```python
from build123d import *

# Parameters (mm, degrees)
MODEL_R                 = 1.5
SALIENTE_EXTRUIR1_DEPTH = 3


with BuildPart() as part:
    # Model → Saliente-Extruir1 (new body)
    with BuildSketch(Plane.XY):
        with BuildLine():
            Line((213.25077615, 152.428489513), (213.25077615, 188.428489513))
            ThreePointArc((213.25077615, 188.428489513), (208.75077615, 192.928489513), (204.25077615, 188.428489513))
            Line((204.25077615, 188.428489513), (204.25077615, 152.428489513))
            ThreePointArc((204.25077615, 152.428489513), (208.75077615, 147.928489513), (213.25077615, 152.428489513))
        make_face()
        with Locations((208.75077615, 179.428489513)):
            Circle(MODEL_R, mode=Mode.SUBTRACT)
        with Locations((208.75077615, 188.428489513)):
            Circle(MODEL_R, mode=Mode.SUBTRACT)
        with Locations((208.75077615, 152.428489513)):
            Circle(MODEL_R, mode=Mode.SUBTRACT)
        with Locations((208.75077615, 161.428489513)):
            Circle(MODEL_R, mode=Mode.SUBTRACT)
        with Locations((208.75077615, 170.428489513)):
            Circle(MODEL_R, mode=Mode.SUBTRACT)
    extrude(amount=SALIENTE_EXTRUIR1_DEPTH)


solid = part.part
```
For this review, take the finished solid that the model builds, in its own axes (mm). Give positions to 0.01 mm unless a question says otherwise; leave off trailing zeros. Write each loop counter-clockwise with the first axis right and the second up, starting at its lowest first coordinate (ties: lowest second). Pieces come first, ordered by that corner, then holes. Notation, with made-up numbers: M 71.25,64.5 L 128.25,64.5 A34 ccw 128.25,96.5 Z; hole C 62,72 d9. An arc over 180 degrees is marked long. One line per item, written item: value.
1) Take a section at C-C, the plane z = 1.45. Write out the cut boundary in (x, y), then the cut area to 3 significant figures.
Results are:
outline: M 204.25,152.43 A4.5 ccw 213.25,152.43 L 213.25,188.43 A4.5 ccw 204.25,188.43 Z; hole C 208.75,152.43 d3; hole C 208.75,161.43 d3; hole C 208.75,170.43 d3; hole C 208.75,179.43 d3; hole C 208.75,188.43 d3
area: 352 mm²
2) Take a section at B-B, the plane y = 153. Write out the cut boundary in (x, z).
Results are:
outline: M 204.25,0 L 207.36,0 L 207.36,3 L 204.25,3 Z; M 210.14,0 L 213.25,0 L 213.25,3 L 210.14,3 Z
3) For line 1 (X direction, y = 152.5, z = 0.2); line 2 (Y direction, x = 209, z = 0.4); line 3 (X direction, y = 160.5, z = 2.55), list the stretches that pass through material, from the lowest coordinate up. Write a range as from..to.
Results are:
line 1: x = 204.25..207.25, 210.25..213.25
line 2: y = 147.94..150.95, 153.91..159.95, 162.91..168.95, 171.91..177.95, 180.91..186.95, 189.91..192.92
line 3: x = 204.25..207.57, 209.93..213.25
4) The part is to be moulded in two halves that separate along X. For faces 1 (the flat face through (213.251, 170, 1)), 2 (the cylindrical face through (208.85, 192.927, 1.479)), 3 (the cylindrical face through (208.556, 189.916, 1.479)), say which applies: +X half, -X half, draft (parallel to the pull), parting line (faces both ways), or undercut.
Results are:
face 1: +X half
face 2: parting line
face 3: undercut
5) Take a section at D-D, the plane x = 205. Write out the cut boundary in (y, z), then the cut area to 3 significant figures.
Results are:
outline: M 149.94,0 L 190.91,0 L 190.91,3 L 149.94,3 Z
area: 123 mm²
6) Take a section at A-A, the plane x = 208. Write out the cut boundary in (y, z), then the cut area to 3 significant figures.
Results are:
outline: M 147.99,0 L 151.13,0 L 151.13,3 L 147.99,3 Z; M 153.73,0 L 160.13,0 L 160.13,3 L 153.73,3 Z; M 162.73,0 L 169.13,0 L 169.13,3 L 162.73,3 Z; M 171.73,0 L 178.13,0 L 178.13,3 L 171.73,3 Z; M 180.73,0 L 187.13,0 L 187.13,3 L 180.73,3 Z; M 189.73,0 L 192.87,0 L 192.87,3 L 189.73,3 Z
area: 95.7 mm²
